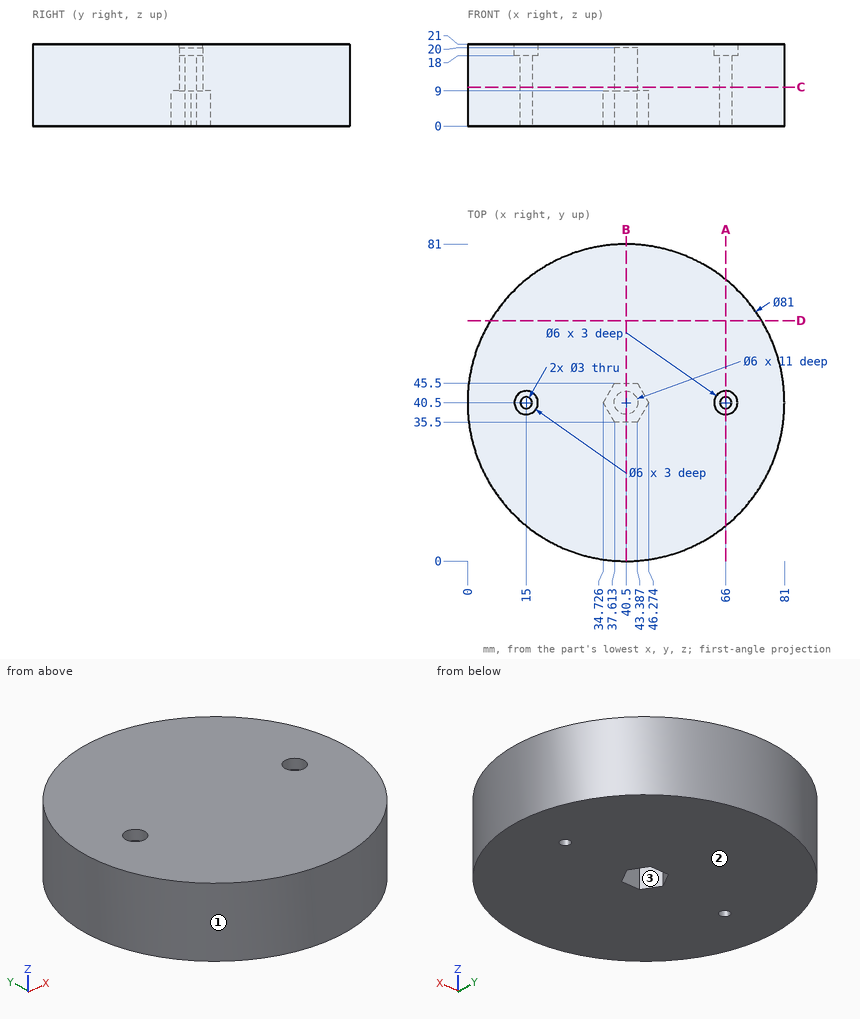
Part print with two shaded views. Sizes in mm from the minimum x, y, z corner. Coordinates: 2 decimals unless noted, no trailing zeros. Write each loop counter-clockwise with the first axis right and the second up, starting at its lowest first coordinate (ties: lowest second). Pieces come first, ordered by that corner, then holes. Notation, with made-up numbers: (76, 45.5) - (113, 45.5) arc R18 cw to (113, 69.5) - close; hole circle Ø2 at (86, -3.75). An arc over 180 degrees is marked (long way). One line per item, written item: value. Start each with the question number.
1. Slice it at A-A (x = 66). Write the cut outline in (y, z) (1 decimal), plus the area to 3 significant figures.
2. Slice it at B-B (x = 40.5). Write the cut outline in (y, z).
3. Mould opens along Y. For the marked faces 1, 2 and 3 say: released by +Y, released by -Y, zero draft, split by the parting line, or undercut.
4. Slice it at D-D (y = 61.5). Write the cut outline in (x, z).
5. Probe line 1 (X direction, y = 41, z = 13.75) (1 decimal); line 2 (Y direction, x = 66, z = 7) (1 decimal); line 3 (Y direction, x = 43.5, z = 3.25) (1 decimal). List the from-to ranges inside material, lowest first. Write a range as from..to.
6. Slice it at C-C (z = 10). Write the cut outline in (x, y).
7. Flat gauge pins, fed straight in: pin 1 (6 mm diameter, centred on x = 35.5, y = 11, fed in from -Z); pin 2 (1.5 mm diameter, centred on y = 55.5, z = 17.5, fed in from -X); pin 3 (2 mm diameter, centred on x = 56, z = 6.5, fed in from -Y) (1 decimal); pin 4 (5 mm diameter, centred on y = 68.5, z = 14.5, fed in from +X) (1 decimal). Where does each tip first touch, or does it go through?
Answers below:
1. outline: (9, 0) - (39, 0) - (39, 18) - (37.5, 18) - (37.5, 21) - (9, 21) - close; (42, 0) - (72, 0) - (72, 21) - (43.5, 21) - (43.5, 18) - (42, 18) - close
1. area: 1,250 mm^2
2. outline: (0, 0) - (35.5, 0) - (35.5, 9) - (37.5, 9) - (37.5, 20) - (43.5, 20) - (43.5, 9) - (45.5, 9) - (45.5, 0) - (81, 0) - (81, 21) - (0, 21) - close
3. face 1: split by the parting line
3. face 2: zero draft
3. face 3: undercut
4. outline: (5.87, 0) - (75.13, 0) - (75.13, 21) - (5.87, 21) - close
5. line 1: x = 0..13.6, 16.4..37.5, 43.5..64.6, 67.4..81
5. line 2: y = 9..39, 42..72
5. line 3: y = 0.1..35.7, 45.3..80.9
6. outline: circle Ø81 at (40.5, 40.5); hole circle Ø3 at (15, 40.5); hole circle Ø6 at (40.5, 40.5); hole circle Ø3 at (66, 40.5)
7. pin 1: stops at z = 0
7. pin 2: stops at x = 2.59
7. pin 3: stops at y = 2.7
7. pin 4: stops at x = 72
